Could you check a few things on this model? Use its own coordinates, in mm. A direction names the side the tool comes from. Give positions to 0.01 mm unless a question says otherwise; leave off trailing zeros. Loops run counter-clockwise (first coordinate to the right, second up) from the corner with the lowest first, then second, coordinate; pieces in that order, holes last.
1. Thinking about a two-plate mould opening in X: for faces 4 (the flat face through (1, 1, -1.6)), 5 (the cylindrical face through (2.015, 1.525, 11.789)), 6 (the flat face through (5.2, 1, 5)), which applies, +X half, -X half, draft (parallel to the pull), parting line (faces both ways), or undercut?
2. I need wall thicknesses on line 1 along Z through (x, y) = (2.85, 1.45); line 2 along X through (y, z) = (1.15, -0.25); line 3 along Y through (x, z) = (1.85, 11.25). Which ranges of each line are inside material? Lowest first, please.
3. Imagine slicing it at B-B (x = 3.3). List the corners of the cut face in (y, z) for me.
4. For faces 1 (the flat face through (3, 1, 11)), 2 (the cylindrical face through (3.305, 1.756, -0.789)), 3 (the flat face through (1, 1, 12.6)), which set-ups out of +Z, -Z, +X, -X, +Y, -Y let a thin tool reach every point of the face, with its end or its side?
5. Imagine slicing it at D-D (y = 0.4). List the corners of the cut face in (x, z) for me, plus the area to 3 significant figures.
6. Imagine slicing it at A-A (y = 1.3). List the corners of the cut face in (x, z) for me, plus the area to 3 significant figures.
7. Imagine slicing it at C-C (x = 1.3). List the corners of the cut face in (y, z) for me.
```python
from build123d import *

# Parameters (mm, degrees)
F0_W     = 5.2
F0_H     = 2.6
F1_DEPTH = 11
F2_R     = 0.75
F3_DEPTH = 1.6
F4_R     = 0.75
F5_DEPTH = 1.6


with BuildPart() as f1:
    # F0 (on Top) → F1 (new body)
    with BuildSketch(Plane.XY):
        with Locations((2.6, 1.3)):
            Rectangle(F0_W, F0_H)
    extrude(amount=F1_DEPTH)

    # F2 (on face) → F3 (join)
    with BuildSketch(Plane.XY.offset(11)):
        with Locations((1.3, 1.3)):
            Circle(F2_R)
        with Locations((3.9, 1.3)):
            Circle(F2_R)
    extrude(amount=F3_DEPTH)

    # F4 (on face) → F5 (join)
    with BuildSketch(Plane(origin=(0, 0, 0), x_dir=(1, 0, 0), z_dir=(0, 0, -1))):
        with Locations((1.3, -1.3)):
            Circle(F4_R)
        with Locations((3.9, -1.3)):
            Circle(F4_R)
    extrude(amount=F5_DEPTH)


solid = f1.part
```
Derived:
1. face 4: draft
1. face 5: undercut
1. face 6: +X half
2. line 1: z = 0 to 11
2. line 2: x = 0.57 to 2.03, 3.17 to 4.63
2. line 3: y = 0.79 to 1.81
3. outline: (0, 0) - (0.85, 0) - (0.85, -1.6) - (1.75, -1.6) - (1.75, 0) - (2.6, 0) - (2.6, 11) - (1.75, 11) - (1.75, 12.6) - (0.85, 12.6) - (0.85, 11) - (0, 11) - close
4. face 1: +Z
4. face 2: -Z
4. face 3: +Z, +X, -X, +Y, -Y
5. outline: (0, 0) - (5.2, 0) - (5.2, 11) - (0, 11) - close
5. area: 57.2 mm2
6. outline: (0, 0) - (0.55, 0) - (0.55, -1.6) - (2.05, -1.6) - (2.05, 0) - (3.15, 0) - (3.15, -1.6) - (4.65, -1.6) - (4.65, 0) - (5.2, 0) - (5.2, 11) - (4.65, 11) - (4.65, 12.6) - (3.15, 12.6) - (3.15, 11) - (2.05, 11) - (2.05, 12.6) - (0.55, 12.6) - (0.55, 11) - (0, 11) - close
6. area: 66.8 mm2
7. outline: (0, 0) - (0.55, 0) - (0.55, -1.6) - (2.05, -1.6) - (2.05, 0) - (2.6, 0) - (2.6, 11) - (2.05, 11) - (2.05, 12.6) - (0.55, 12.6) - (0.55, 11) - (0, 11) - close
